CAD build for the part. Positions are in the model's coordinates, mm. Face numbers are marked on the shaded views. A direction names the side the tool comes from. Round coordinates to 2 decimals unless told otherwise and drop trailing zeros. Loops run counter-clockwise (first coordinate to the right, second up) from the corner with the lowest first, then second, coordinate; pieces in that order, holes last.
Autodesk Inventor part; units mm, degrees
ref_plane "YZ Plane" through (0, 0, 0) normal (1, 0, 0) x (0, 1, 0)
ref_plane "XZ Plane" through (0, 0, 0) normal (0, 1, 0) x (-1, 0, 0)
ref_plane "XY Plane" through (0, 0, 0) normal (0, 0, 1) x (1, 0, 0)
sketch "Szkic1" plane through (0, 0, 0) normal (0, 1, 0) x (-1, 0, 0)
  line L0 (40, -25) -> (-40, -25)
  line L1 (-40, -25) -> (-40, 25)
  line L2 (-40, 25) -> (40, 25)
  line L3 (40, 25) -> (40, -25)
  point P0 (0, 0)
  dimension "d0" = 80
  dimension "d1" = 50
extrude "Wyciągnięcie proste1" add sketch "Szkic1" along normal blind 8
sketch "Szkic2" plane through (0, 8, 0) normal (0, 1, 0) x (1, 0, 0)
  line L0 (40, -25) -> (40, 25)
  line L1 (-40, -20) -> (40, -20)
  line L2 (40, -20) -> (40, 20)
  line L3 (40, 20) -> (-40, 20)
  line L4 (-40, 20) -> (-40, -20)
  line L5 (-40, -20) -> (40, 20) construction
  line L6 (40, -20) -> (-40, 20) construction
  point P0 (0, 0)
  dimension "d4" = 40
extrude "Wyciągnięcie proste2" add sketch "Szkic2" along normal blind 42
sketch "Szkic3" plane through (-40, 8, 20) normal (0, 0, 1) x (1, 0, 0)
  line L0 (0, 0) -> (0, 42)
  line L1 (0, 0) -> (0, 7)
  circle A0 centre (65, 27) radius 15
  line L2 (80, 0) -> (80, 42)
  line L3 (0, 42) -> (80, 42)
  line L4 (0, 7) -> (57.5352, 40.0106)
  point P0 (40, -8)
  point P1 (65, 42)
  point P2 (80, 27)
  dimension "d8" = 30
  dimension "d7" = 7
extrude "Wyciągnięcie proste3" cut sketch "Szkic3" against normal through all contours L0 L3 A0 L4 | L3 L2 A0
sketch "Szkic4" plane through (40, 0, 25) normal (1, 0, 0) x (0, 0, -1)
  line L0 (12.5, 20) -> (37.5, 20)
  line L1 (37.5, 20) -> (37.5, 50)
  line L2 (37.5, 50) -> (12.5, 50)
  line L3 (12.5, 50) -> (12.5, 20)
  line L4 (12.5, 20) -> (37.5, 50) construction
  line L5 (37.5, 20) -> (12.5, 50) construction
  line L6 (0, 0) -> (50, 0)
  point P0 (25, 0)
  point P1 (25, 35)
  dimension "d11" = 25
  dimension "d12" = 30
  dimension "d13" = 20
sketch "Szkic5" plane through (-40, 8, 20) normal (0, 0, 1) x (1, 0, 0)
  arc A0 (80, 27) -> (57.5352, 40.0106) centre (65, 27) ccw
  point P0 (40, -8)
extrude "Wyciągnięcie proste4" cut sketch "Szkic4" against normal through all
sketch "Szkic6" plane through (40, 20, 12.5) normal (0, 1, 0) x (1, 0, 0)
  line L0 (-55, 18.5) -> (-80, 18.5)
  line L1 (-80, 18.5) -> (-80, 6.5)
  line L2 (-80, 6.5) -> (-55, 6.5)
  line L3 (-55, 6.5) -> (-55, 18.5)
  line L4 (-55, 18.5) -> (-80, 6.5) construction
  line L5 (-80, 18.5) -> (-55, 6.5) construction
  line L6 (0, 25) -> (0, 0)
  point P0 (-40, 12.5)
  point P1 (-67.5, 12.5)
  point P2 (-55, 12.5)
  dimension "d16" = 25
  dimension "d17" = 55
  dimension "d18" = 12
extrude "Wyciągnięcie proste5" cut sketch "Szkic6" against normal blind 4
hole "Otwór1" at (25, 35, 20) direction (0, 0, -1) diameter 15 end through all
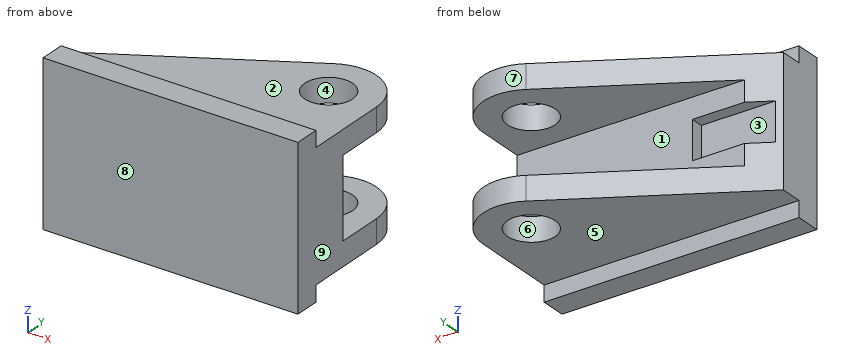
Item 1: Cut at B-B, the plane z = -16.5. Give the cut face in (x, y).
Answers follow:
outline: (-40, 0) - (40, 0) - (40, 35) arc R15 ccw to (17.54, 48.01) - (-40, 15) - close; hole circle Ø15 at (25, 35)
Item 2: Probe line 1 (Y direction, x = 25, z = -14.5); line 2 (Z direction, x = 16, y = 23); line 3 (X direction, y = 35, z = 17.5). List the from-to ranges inside material, lowest first.
Answers follow:
line 1: y = 0 to 27.5, 42.5 to 50
line 2: z = -20 to -12.5, 12.5 to 20
line 3: x = -5.14 to 17.5, 32.5 to 40
Item 3: Flat gauge pins, fed straight in: P1, Ø10, axis at x = 30.5, y = 14, coming from the -Z side; P2, Ø4, axis at x = -3, z = 22.5, coming from the +Y side; P3, Ø6, axis at x = -29, z = -0.5, coming from the +Y side. Where does each tip first touch, or does it go through?
Answers follow:
P1: stops at z = -20
P2: stops at y = 8
P3: stops at y = 16
Item 4: Cut at D-D, the plane z = -4.5. Give the cut face in (x, y).
Answers follow:
outline: (-40, 0) - (40, 0) - (40, 20) - (-15, 20) - (-15, 16) - (-38.26, 16) - (-40, 15) - close
Item 5: Two-plate mould, pull along Y, no slides. Class the marked faces 6, 7, 8 and 9: released by +Y, released by -Y, zero draft, split by the parting line, or undercut.
Answers follow:
face 6: undercut
face 7: released by +Y
face 8: released by -Y
face 9: zero draft
Item 6: Cut at A-A, the plane x = 25. Give the cut face in (y, z), plus the area to 4 significant figures.
Answers follow:
outline: (0, -25) - (8, -25) - (8, -20) - (27.5, -20) - (27.5, -12.5) - (20, -12.5) - (20, 12.5) - (27.5, 12.5) - (27.5, 20) - (8, 20) - (8, 25) - (0, 25) - close; (42.5, -20) - (50, -20) - (50, -12.5) - (42.5, -12.5) - close; (42.5, 12.5) - (50, 12.5) - (50, 20) - (42.5, 20) - close
area: 1,105 mm2
Item 7: 3-axis set-ups, long thin cutter, end or side, ignore diameter. For the marked faces 1, 2, 3, 4 and 5: which of +Z, -Z, +X, -X, +Y, -Y reach the whole face in a straight line?
Answers follow:
face 1: +X, -X, +Y
face 2: +Z, +X, -X, +Y
face 3: -X, +Y
face 4: +Z, -Z
face 5: -Z, +X, -X, +Y
Item 8: Cut at C-C, the plane y = 40. Give the cut face in (x, z).
Answers follow:
outline: (3.57, -20) - (19.41, -20) - (19.41, -12.5) - (3.57, -12.5) - close; (3.57, 12.5) - (19.41, 12.5) - (19.41, 20) - (3.57, 20) - close; (30.59, -20) - (39.14, -20) - (39.14, -12.5) - (30.59, -12.5) - close; (30.59, 12.5) - (39.14, 12.5) - (39.14, 20) - (30.59, 20) - close
